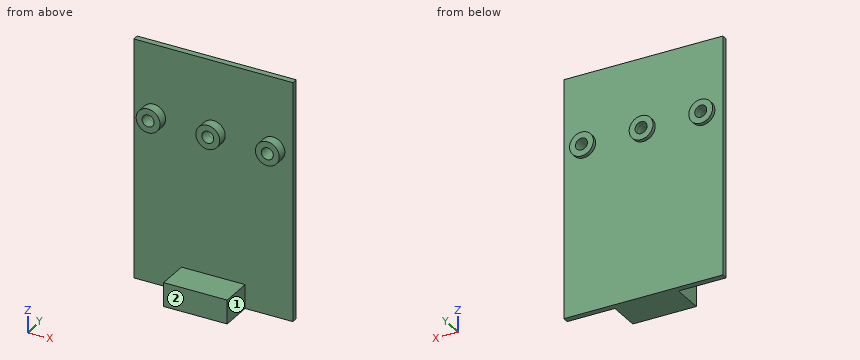
from build123d import *

# Parameters (mm, degrees)
F0_W     = 400
F0_H     = 600
F1_DEPTH = 15
F2_R     = 30
F2_R_2   = 15
F3_DEPTH = 25
F4_DEPTH = 25.001
F5_W     = 160
F5_H     = 60
F6_DEPTH = 80


with BuildPart() as f1:
    # F0 (on Front) → F1 (new body)
    with BuildSketch(Plane.XZ):
        Rectangle(F0_W, F0_H)
    extrude(amount=-F1_DEPTH)

    # F2 (on face) → F3 (join, symmetric)
    with BuildSketch(Plane.XZ):
        with Locations((-150, 120)):
            Circle(F2_R)
        with Locations((-150, 120)):
            Circle(F2_R_2, mode=Mode.SUBTRACT)
        with Locations((0, 120)):
            Circle(F2_R)
        with Locations((0, 120)):
            Circle(F2_R_2, mode=Mode.SUBTRACT)
        with Locations((150, 120)):
            Circle(F2_R)
        with Locations((150, 120)):
            Circle(F2_R_2, mode=Mode.SUBTRACT)
    extrude(amount=F3_DEPTH, both=True)

    # F4 (cut, through all): faces of the model
    f4_faces = [f1.faces().sort_by_distance(p)[0] for p in [
        (150, 0, 120),
        (0, 0, 120),
        (-150, 0, 120),
    ]]
    extrude(f4_faces, amount=-F4_DEPTH, mode=Mode.SUBTRACT)

    # F5 (on face) → F6 (join)
    with BuildSketch(Plane.XZ):
        with Locations((0, -270)):
            Rectangle(F5_W, F5_H)
    extrude(amount=F6_DEPTH)


solid = f1.part
Here's how the part is built. I have some questions about the finished solid (model axes, mm). Face numbers are marked on the shaded views. A direction names the side the tool comes from. Coordinates: 2 decimals unless noted, no trailing zeros. Loops run counter-clockwise (first coordinate to the right, second up) from the corner with the lowest first, then second, coordinate; pieces in that order, holes last. Notation, with made-up numbers: (59, 83.25) -> (96, 83.25) arc R26 cw to (96, 106.25) -> close; hole circle Ø2 at (15, 41). An arc over 180 degrees is marked (long way). Use one line per item in the form item = value. Start each with the question number.
(1) Please list where these lines run through material, in increasing order: line 1 along Z through (x, y) = (-150, -12); line 2 along Y through (x, z) = (-59.5, -193); line 3 along Z through (x, y) = (-150, 4.25).
(2) If we section it at C-C (x = 0): Please give me the cut outline in (y, z), then the cut area to 3 significant figures.
(3) If we section it at B-B (z = 120): Give the number of separate pieces and of enclosed holes in the cut face, then the cut area to 3 significant figures.
(4) If we section it at A-A (x = -150): Please give me the cut outline in (y, z).
(5) On a 3-axis mill with a long thin cutter (end or side, diameter ignored), from which of +Z, -Z, +X, -X, +Y, -Y can I reach the whole of each face in a straight line? I mean the marked faces 1 and 2. Say none if no direction works.
(6) Will these pins go through, and if not, where does the flat tip stop? pin 1 (18 mm diameter, centred on y = -29.5, z = -280, fed in from +X); pin 2 (6 mm diameter, centred on x = 131, y = -20.5, fed in from -Z); pin 3 (18 mm diameter, centred on y = -49.5, z = -279.5, fed in from -X).
(7) If we section it at D-D (y = -39): Please give me the cut outline in (x, z), then the cut area to 3 significant figures.
Verdict:
q1.line_1 = 90 to 105, 135 to 150
q1.line_2 = 0 to 15
q1.line_3 = -300 to 105, 135 to 300
q2.outline = (-80, -300) -> (15, -300) -> (15, 90) -> (25, 90) -> (25, 105) -> (-25, 105) -> (-25, 90) -> (0, 90) -> (0, -240) -> (-80, -240) -> close; (-25, 135) -> (25, 135) -> (25, 150) -> (15, 150) -> (15, 300) -> (0, 300) -> (0, 150) -> (-25, 150) -> close
q2.area = 14,400 mm²
q3.separate_pieces = 4
q3.enclosed_holes = 0
q3.area = 7,800 mm²
q4.outline = (-25, 90) -> (0, 90) -> (0, -300) -> (15, -300) -> (15, 90) -> (25, 90) -> (25, 105) -> (-25, 105) -> close; (-25, 135) -> (25, 135) -> (25, 150) -> (15, 150) -> (15, 300) -> (0, 300) -> (0, 150) -> (-25, 150) -> close
q5.face_1 = +Z, -Z, +X, -Y
q5.face_2 = +Z, -Z, +X, -X, -Y
q6.pin_1 = 80
q6.pin_2 = 94.62
q6.pin_3 = -80
q7.outline = (-80, -300) -> (80, -300) -> (80, -240) -> (-80, -240) -> close
q7.area = 9,600 mm²
